```python
from build123d import *

# Parameters (mm, degrees)
F1_DEPTH = 43.18
F3_R     = 9.525
F4_DEPTH = 53.34
F5_R     = 1.5875
F6_DEPTH = 57.15


with BuildPart() as f1:
    # F0 (on Front) → F1 (new body)
    with BuildSketch(Plane.XZ):
        with BuildLine():
            Line((0, 62.539058), (0, 0))
            Line((0, 0), (304.765889, 4.559934))
            Line((304.765889, 4.559934), (304.636415, 13.213416))
            ThreePointArc((304.636415, 13.213416), (302.426417, 17.933889), (297.427606, 19.409977))
            ThreePointArc((297.427606, 19.409977), (149.599987, 21.769594), (9.232421, 68.197163))
            ThreePointArc((9.232421, 68.197163), (3.031934, 67.953201), (0, 62.539058))
        make_face()
    extrude(amount=-F1_DEPTH)

    # F3 (on face) → F4 (cut)
    with BuildSketch(Plane(origin=(0, 0, 0), x_dir=(0, -1, 0), z_dir=(-1, 0, 0))):
        with Locations((-21.59, 31.269529)):
            Circle(F3_R)
    extrude(amount=-F4_DEPTH, mode=Mode.SUBTRACT)

    # F5 (on face) → F6 (cut)
    with BuildSketch(Plane.XZ):
        with Locations((17.067824, 10.321916)):
            Circle(F5_R)
        with Locations((293.850511, 10.321916)):
            Circle(F5_R)
    extrude(amount=-F6_DEPTH, mode=Mode.SUBTRACT)


solid = f1.part
```
Verification items for the finished model (mm, model axes). A direction names the side the tool comes from. Give positions to 0.01 mm unless a question says otherwise; leave off trailing zeros. Loops run counter-clockwise (first coordinate to the right, second up) from the corner with the lowest first, then second, coordinate; pieces in that order, holes last.
1. Section check C-C, the plane x = 78.5. Enter the section's corners in (y, z), then the cut area to 3 significant figures.
2. Mould release check, pull along X, two halves, no side actions. Record for faces 3 (the cylindrical face through (3.11, 21.29, 68)), 4 (the flat face through (0, 11.7, 31.7)), 5 (the cylindrical face through (151.649, 21.288, 21.427)): released by +X, released by -X, zero draft, split by the parting line, or undercut.
3. Section check A-A, the plane y = 35. Count the separate pieces of the cut face and the enclosed holes in it, then the cut area to 3 significant figures.
4. Set-up check for faces 1 (the flat face through (116, 43.18, 20)), 2 (the flat face through (53.34, 22, 31)): record each of +Z, -Z, +X, -X, +Y, -Y from which the full face is reachable in a straight line by a thin tool's end or side.
5. Thickness scan on line 1 (X direction, y = 38, z = 10); line 2 (X direction, y = 14.5, z = 9); line 3 (Z direction, x = 17, y = 21.59). Record the ranges inside material, lowest first.
6. Go/stop test with flat-tipped pins: pin 1 Ø2 at (x, y) = (199, 8.5) entering from -Z; pin 2 Ø3 at (x, y) = (185.5, 9) entering from -Z; pin 3 Ø5 at (x, y) = (255.5, 14.5) entering from -Z. Record where each tip stops, or that it passes through.
7. Section check D-D, the plane x = 228. Enter the section's corners in (y, z), then the cut area to 3 significant figures.
Geometry says:
1. outline: (0, 1.17) - (43.18, 1.17) - (43.18, 39.37) - (0, 39.37) - close
1. area: 1,650 mm2
2. face 3: split by the parting line
2. face 4: released by -X
2. face 5: undercut
3. separate pieces: 1
3. enclosed holes: 2
3. area: 8,300 mm2
4. face 1: +Z, -Z, +X, -X, +Y
4. face 2: -X
5. line 1: x = 0 to 15.51, 18.62 to 292.3, 295.41 to 304.68
5. line 2: x = 0 to 16.19, 17.95 to 292.97, 294.73 to 304.7
5. line 3: z = 0.25 to 8.74, 11.91 to 21.74, 40.79 to 64.33
6. pin 1: stops at z = 2.96
6. pin 2: stops at z = 2.75
6. pin 3: stops at z = 3.79
7. outline: (0, 3.41) - (43.18, 3.41) - (43.18, 14.92) - (0, 14.92) - close
7. area: 497 mm2
